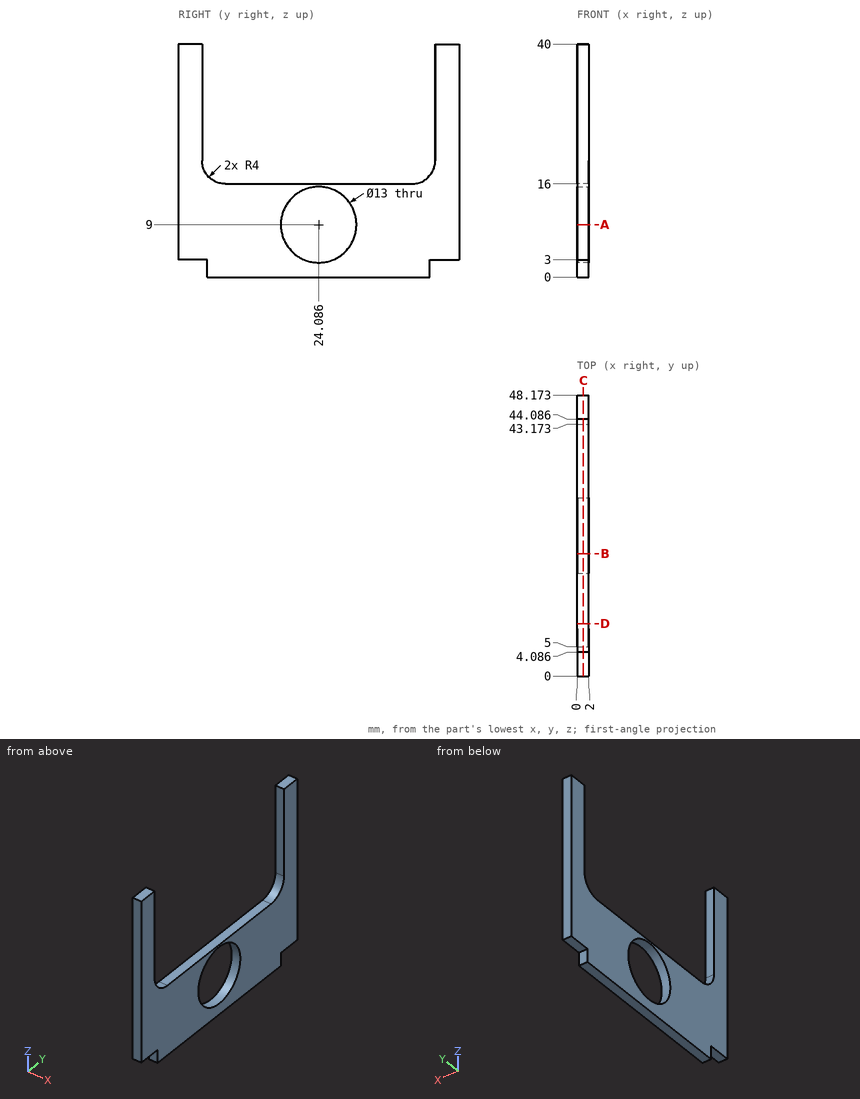
Geometry: see drawing. Coordinates: mm, zero at the bounding-box minimum. Give positions to 0.01 mm unless a question says otherwise; leave off trailing zeros. Order: outer loops, then holes, each group sorted by start corner. A loop starts at its lowest first (then second) coordinate and runs counter-clockwise, first axis right, second up.
1. Line query: probe 1 along Z at (x, y) = (1.35, 24); probe 2 along Y at (x, z) = (0.55, 21); probe 3 along Y at (x, z) = (0.4, 9). Output: solid intervals per line, ascending.
Computed:
probe 1: z = 0 to 2.5, 15.5 to 16
probe 2: y = 0 to 4.09, 44.09 to 48.17
probe 3: y = 0 to 17.59, 30.59 to 48.17
2. Cut plane B-B (y = 21). Return loops of the section in (x, z).
Computed:
outline: (0, 0) - (2, 0) - (2, 3.28) - (0, 3.28) - close; (0, 14.72) - (2, 14.72) - (2, 16) - (0, 16) - close
3. Cut plane C-C (x = 1.1). Return loops of the section in (y, z).
Computed:
outline: (0, 3) - (5, 3) - (5, 0) - (43.17, 0) - (43.17, 3) - (48.17, 3) - (48.17, 40) - (44.09, 40) - (44.09, 20) arc R4 cw to (40.09, 16) - (8.09, 16) arc R4 cw to (4.09, 20) - (4.09, 40) - (0, 40) - close; hole circle Ø13 at (24.09, 9)
4. Pin query (flat end, axial travel): pin 1 Ø0.6 at (x, y) = (1.5, 45.5) entering from -Z; pin 2 Ø8 at (y, z) = (24.09, 9) entering from +X; pin 3 Ø1 at (x, y) = (1, 26.5) entering from +Z. Return the tip coordinate at first contact, or that it passes through.
Computed:
pin 1: stops at z = 3
pin 2: passes through
pin 3: stops at z = 16
5. Cut plane A-A (z = 9). Return loops of the section in (x, y).
Computed:
outline: (0, 0) - (2, 0) - (2, 17.59) - (0, 17.59) - close; (0, 30.59) - (2, 30.59) - (2, 48.17) - (0, 48.17) - close
6. Cut plane D-D (y = 9). Return loops of the section in (x, z).
Computed:
outline: (0, 0) - (2, 0) - (2, 16) - (0, 16) - close
